from build123d import *

# Parameters (mm, degrees)
BOSS_EXTRUDE1_DEPTH     = 10
CUT_EXTRUDE1_DEPTH      = 116.537872579
CUT_EXTRUDE1_DEPTH_BACK = 116.537872579
SKETCH2_R               = 2
SKETCH2_W               = 28.5
SKETCH2_H               = 40
SKETCH5_R               = 2
CUT_EXTRUDE2_DEPTH      = 152.973681932
SKETCH6_R               = 2
BOSS_EXTRUDE2_DEPTH     = 40
SKETCH7_W               = 79.874147132
SKETCH7_H               = 7.5
SKETCH7_W_2             = 36.93403835
SKETCH7_H_2             = 7.021862101
SKETCH7_W_3             = 1.5
SKETCH7_H_3             = 37.978137899
BOSS_EXTRUDE3_DEPTH     = 30
CUT_EXTRUDE3_DEPTH      = 122.856472951
CUT_EXTRUDE3_DEPTH_BACK = 122.856472951
SKETCH8_R               = 7.5


with BuildPart() as part:
    # Sketch1 → Boss-Extrude1 (new body)
    with BuildSketch(Plane(origin=(0, 0, 0), x_dir=(1, 0, 0), z_dir=(0, 1, 0))):
        Polygon((30, 0), (-30, 0), (-30, 45), (-57, 45), (-57, 100), (57, 100), (57, 45), (30, 45), align=None)
    extrude(amount=BOSS_EXTRUDE1_DEPTH)

    # Sketch2 → Cut-Extrude1 (cut, two sides: drawn at the far end of the back side and taken through both)
    with BuildSketch(Plane(origin=(0, 10, 0), x_dir=(1, 0, 0), z_dir=(0, 1, 0)).offset(-CUT_EXTRUDE1_DEPTH_BACK)):
        with Locations(Location((-52, 95, 0), (0, 0, 270))):
            Circle(SKETCH2_R)
        with Locations(Location((52, 95, 0), (0, 0, 270))):
            Circle(SKETCH2_R)
        with Locations(Location((-25, 5, 0), (0, 0, 270))):
            Circle(SKETCH2_R)
        with Locations(Location((25, 5, 0), (0, 0, 270))):
            Circle(SKETCH2_R)
        with Locations((-41.25, 72.5)):
            Rectangle(SKETCH2_W, SKETCH2_H)
        with Locations((41.25, 72.5)):
            Rectangle(SKETCH2_W, SKETCH2_H)
    extrude(amount=CUT_EXTRUDE1_DEPTH + CUT_EXTRUDE1_DEPTH_BACK, mode=Mode.SUBTRACT)

    # Sketch5 → Cut-Extrude2 (cut, through all)
    with BuildSketch(Plane(origin=(57, 0, 0), x_dir=(0, 0, -1), z_dir=(1, 0, 0))):
        with Locations(Location((55.064404226, 3.5, 0), (0, 0, 180))):
            Circle(SKETCH5_R)
        with Locations(Location((89.935595774, 3.5, 0), (0, 0, 180))):
            Circle(SKETCH5_R)
    extrude(amount=-CUT_EXTRUDE2_DEPTH, mode=Mode.SUBTRACT)

    # Sketch6 → Boss-Extrude2 (add)
    with BuildSketch(Plane(origin=(0, 10, 0), x_dir=(1, 0, 0), z_dir=(0, 1, 0))):
        with Locations(Location((-25, 5, 0), (0, 0, 270))):
            Circle(SKETCH6_R)
        with Locations(Location((25, 5, 0), (0, 0, 270))):
            Circle(SKETCH6_R)
        with Locations(Location((52, 95, 0), (0, 0, 270))):
            Circle(SKETCH6_R)
        with Locations(Location((-52, 95, 0), (0, 0, 270))):
            Circle(SKETCH6_R)
    extrude(amount=-BOSS_EXTRUDE2_DEPTH)

    # Sketch7 → Boss-Extrude3 (add)
    with BuildSketch(Plane.XZ):
        with Locations((0, -96.25)):
            Rectangle(SKETCH7_W, SKETCH7_H)
        with Locations((0, -3.510931051)):
            Rectangle(SKETCH7_W_2, SKETCH7_H_2)
        with Locations((-29.25, -26.010931051)):
            Rectangle(SKETCH7_W_3, SKETCH7_H_3)
        with Locations((29.25, -26.010931051)):
            Rectangle(SKETCH7_W_3, SKETCH7_H_3)
    extrude(amount=BOSS_EXTRUDE3_DEPTH)

    # Sketch8 → Cut-Extrude3 (cut, two sides: drawn at the far end of the back side and taken through both)
    with BuildSketch(Plane(origin=(0, 10, 0), x_dir=(1, 0, 0), z_dir=(0, 1, 0)).offset(-CUT_EXTRUDE3_DEPTH_BACK)):
        with Locations(Location((0, 80.227050859, 0), (0, 0, 270))):
            Circle(SKETCH8_R)
    extrude(amount=CUT_EXTRUDE3_DEPTH + CUT_EXTRUDE3_DEPTH_BACK, mode=Mode.SUBTRACT)


solid = part.part
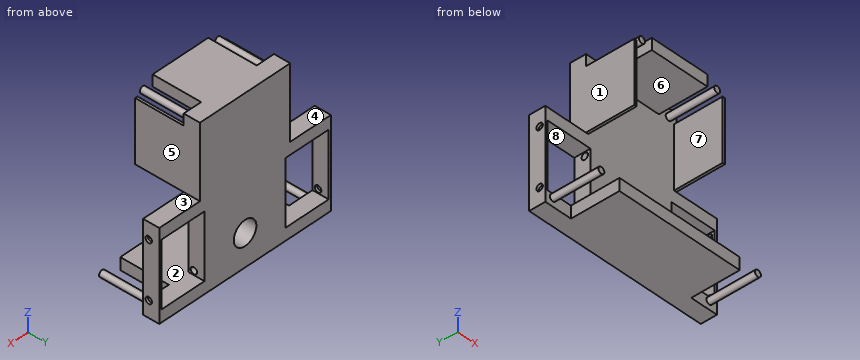
Geometry check sheet. Reference: the model listing, model coordinates, mm. Face numbers are marked on the shaded views. A direction names the side the tool comes from. Give positions to 0.01 mm unless a question says otherwise; leave off trailing zeros. Write each loop counter-clockwise with the first axis right and the second up, starting at its lowest first coordinate (ties: lowest second). Pieces come first, ordered by that corner, then holes.
1) Set-up check for the marked faces 4, 5, 6, 7 and 8: record each of +Z, -Z, +X, -X, +Y, -Y from which the full face is reachable in a straight line by a thin tool's end or side.
Values follow:
face 4: +Z, -X, +Y, -Y
face 5: +Z, +X, +Y, -Y
face 6: -Y
face 7: +Z, -Y
face 8: +Y, -Y
2) Cross-section at B-B (z = -64). Record the boundary of the cut face in (x, y), plus the area to 3 significant figures.
Values follow:
outline: (-57, 0) - (-55.5, 0) - (-55.5, 10) - (-57, 10) - close; (-27, 0) - (27, 0) - (27, 10) - (-27, 10) - close; (55.5, 0) - (57, 0) - (57, 10) - (55.5, 10) - close
area: 570 mm2
3) Cross-section at A-A (x = -47). Record the boundary of the cut face in (y, z), plus the area to 3 significant figures.
Values follow:
outline: (0, -100) - (10, -100) - (10, -92.5) - (0, -92.5) - close; (0, -52.5) - (10, -52.5) - (10, -45) - (0, -45) - close
area: 150 mm2
4) Cross-section at C-C (y = -17). Record the boundary of the cut face in (x, z), plus the area to 3 significant figures.
Values follow:
outline: circle Ø4 at (-52, -95); (-39.94, -100) - (39.94, -100) - (39.94, -92.5) - (-39.94, -92.5) - close; (-30, -45) - (-28.5, -45) - (-28.5, -7.02) - (-30, -7.02) - close; circle Ø4 at (-25, -5); (-18.47, -7.02) - (18.47, -7.02) - (18.47, 0) - (-18.47, 0) - close; circle Ø4 at (25, -5); (28.5, -45) - (30, -45) - (30, -7.02) - (28.5, -7.02) - close; circle Ø4 at (52, -95)
area: 1,020 mm2
5) Go/stop test with flat-tipped pins: pin 1 Ø4 at (x, y) = (-42, -2.5) entering from -Z; pin 2 Ø12 at (x, z) = (14, -32.5) entering from -Y; pin 3 Ø12 at (y, z) = (-1, -12.5) entering from +X; pin 4 Ø20 at (y, z) = (-18.5, -25.5) entering from -X. Record where each tip stops, or that it passes through.
Values follow:
pin 1: passes through
pin 2: stops at y = 0
pin 3: stops at x = 30
pin 4: stops at x = -30
6) Release check for a two-part mould opening along X. For the marked faces 1, 2 and 3 record: released by +X, released by -X, zero draft, split by the parting line, or undercut.
Values follow:
face 1: released by -X
face 2: undercut
face 3: zero draft
7) Thickness scan on line 1 (X direction, y = -20.5, z = -21.5); line 2 (Z direction, x = 37, y = 6.5); line 3 (Z direction, x = -3, y = -11.5). Record the ranges inside material, lowest first.
Values follow:
line 1: x = -30 to -28.5, 28.5 to 30
line 2: z = -100 to -92.5, -52.5 to -45
line 3: z = -100 to -92.5, -7.02 to 0
8) Cross-section at D-D (x = 0). Record the boundary of the cut face in (y, z), plus the area to 3 significant figures.
Values follow:
outline: (-30, -100) - (10, -100) - (10, -87.73) - (0, -87.73) - (0, -92.5) - (-30, -92.5) - close; (-30, -7.02) - (0, -7.02) - (0, -72.73) - (10, -72.73) - (10, 0) - (-30, 0) - close; hole circle Ø4 at (3.5, -89.94); hole circle Ø4 at (3.5, -55.06)
area: 1,260 mm2
